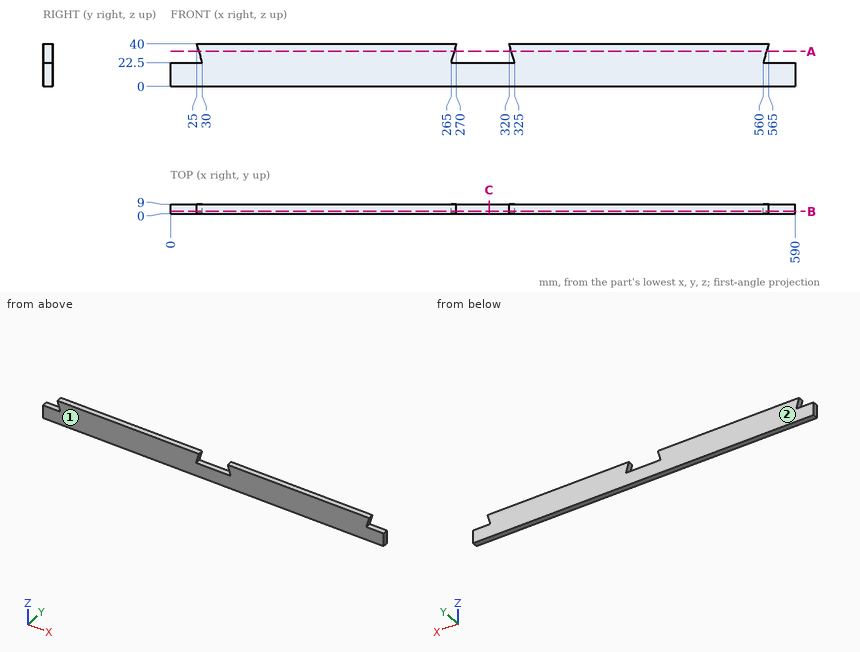
Verification items for this drawing (mm, ordinates from the low corner). Coordinates: 2 decimals unless noted, no trailing zeros. Order: outer loops, then holes, each group sorted by start corner. A loop starts at its lowest first (then second) coordinate and runs counter-clockwise, first axis right, second up.
Q1. Draft check along Y on the marked faces 1 and 2. Enter one of: released by +Y, released by -Y, zero draft, split by the parting line, or undercut.
Reply:
face 1: released by -Y
face 2: released by +Y
Q2. Sectioned sample at A-A on z = 33. Record the cut outline in (x, y), and give its area (3 significant figures).
Reply:
outline: (27, 0) - (268, 0) - (268, 9) - (27, 9) - close; (322, 0) - (563, 0) - (563, 9) - (322, 9) - close
area: 4,340 mm2
Q3. Sectioned sample at C-C on x = 301. Record the cut outline in (y, z), and give its area (4 significant figures).
Reply:
outline: (0, 0) - (9, 0) - (9, 22.5) - (0, 22.5) - close
area: 202.5 mm2
Q4. Thickness scan on probe 1 along Z at (x, y) = (285, 3.75); probe 2 along X at (y, z) = (3.25, 34.5); probe 3 along X at (y, z) = (2.5, 37). Record the ranges inside material, lowest first.
Reply:
probe 1: z = 0 to 22.5
probe 2: x = 26.57 to 268.43, 321.57 to 563.43
probe 3: x = 25.86 to 269.14, 320.86 to 564.14
Q5. Sectioned sample at B-B on y = 2.25. Record the cut outline in (x, z), and give its area (3 significant figures).
Reply:
outline: (0, 0) - (590, 0) - (590, 22.5) - (560, 22.5) - (565, 40) - (320, 40) - (325, 22.5) - (265, 22.5) - (270, 40) - (25, 40) - (30, 22.5) - (0, 22.5) - close
area: 21,700 mm2
Q6. Depth check by flat-ended pin: pin 1 Ø2.5 at (x, y) = (21, 4.5) entering from +Z; pin 2 Ø2 at (y, z) = (7, 29) entering from +X. Enter the tip coordinate at first touch or a pass-through.
Reply:
pin 1: stops at z = 22.5
pin 2: stops at x = 562.14
